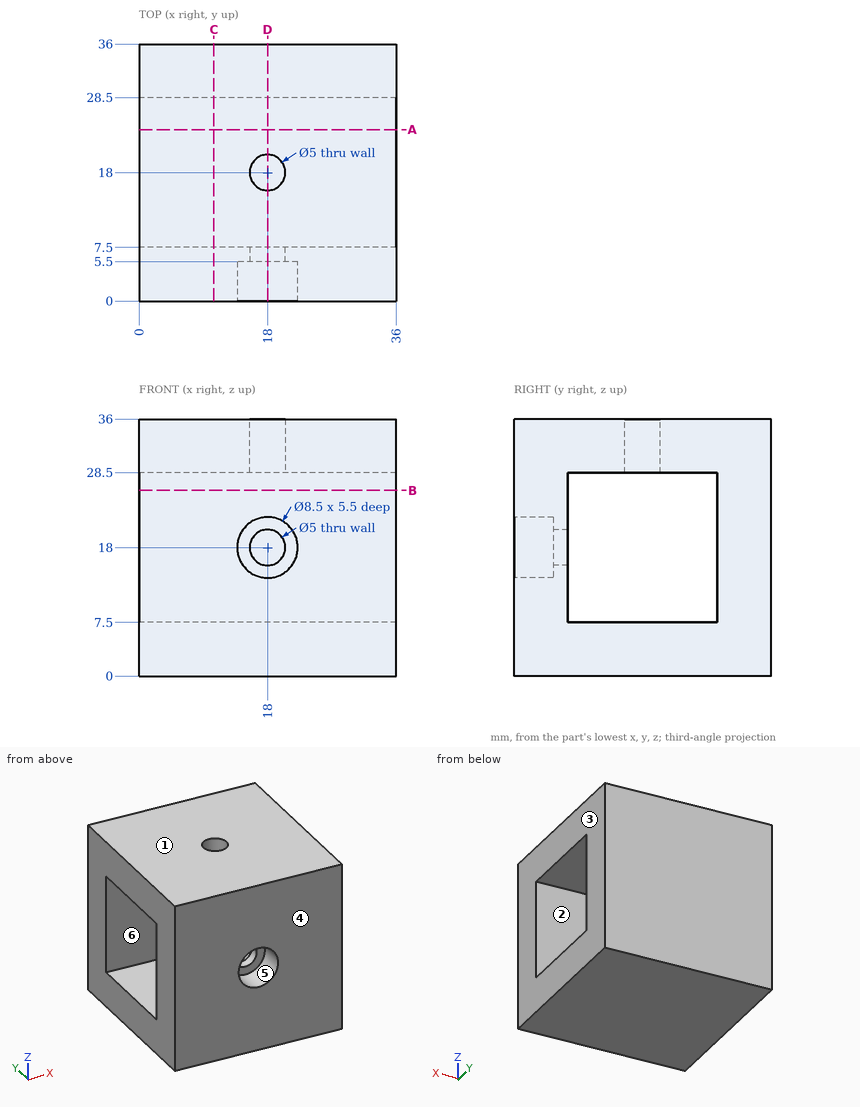
Design review of the part shown in the three views and the two pictorial views. Dimensions are in mm from the part's minimum x, y and z. A direction names the side the tool comes from. Give positions to 0.01 mm unless a question says otherwise; leave off trailing zeros. Write each loop counter-clockwise with the first axis right and the second up, starting at its lowest first coordinate (ties: lowest second). Pieces come first, ordered by that corner, then holes. Notation, with made-up numbers: (-1.75, 50.5) -> (10.25, 50.5) arc R5 ccw to (10.25, 54.5) -> close; hole circle Ø5 at (28.5, 68). An arc over 180 degrees is marked (long way). Answer in a Markdown table with one row per item.
1) Tool access review of the marked faces 4, 5 and 6: name each direction out of +Z, -Z, +X, -X, +Y, -Y from which nothing blocks a thin tool from reaching the whole face with its end or side.
Worked answers:
| item | result |
|---|---|
| face 4 | +Z, -Z, +X, -X, -Y |
| face 5 | -Y |
| face 6 | +X, -X |
2) Mouldability with a two-part tool opening along Z and no side actions: class the marked faces 1, 2 and 3 as +Z half, -Z half, draft (parallel to the pull), parting line (faces both ways), or undercut.
Worked answers:
| item | result |
|---|---|
| face 1 | +Z half |
| face 2 | undercut |
| face 3 | draft |
3) Add section C-C on x = 10.5. State the section outline as (y, z) points.
Worked answers:
| item | result |
|---|---|
| outline | (0, 0) -> (36, 0) -> (36, 36) -> (0, 36) -> close; hole (7.5, 7.5) -> (28.5, 7.5) -> (28.5, 28.5) -> (7.5, 28.5) -> close |
4) For L1, parallel to Z at x = 25, y = 19.5; L2, parallel to Z at x = 18, y = 6.85, list the stretches that pass through material, from the lowest coordinate up. Write a range as [from, to].
Worked answers:
| item | result |
|---|---|
| L1 | [0, 7.5], [28.5, 36] |
| L2 | [0, 15.5], [20.5, 36] |
5) Clearance check with flat-ended pins moving along their axes: P1, Ø3, axis at y = 26.5, z = 7.5, coming from the -X side; P2, Ø3, axis at x = 18, y = 18, coming from the +Z side; P3, Ø7, axis at x = 18.5, z = 18, coming from the -Y side. State where each tip first meets the part, or that it passes through.
Worked answers:
| item | result |
|---|---|
| P1 | x = 0 |
| P2 | z = 7.5 |
| P3 | y = 5.5 |
6) Add section D-D on x = 18. State the section outline as (y, z) points.
Worked answers:
| item | result |
|---|---|
| outline | (0, 0) -> (36, 0) -> (36, 36) -> (20.5, 36) -> (20.5, 28.5) -> (28.5, 28.5) -> (28.5, 7.5) -> (7.5, 7.5) -> (7.5, 15.5) -> (5.5, 15.5) -> (5.5, 13.75) -> (0, 13.75) -> close; (0, 22.25) -> (5.5, 22.25) -> (5.5, 20.5) -> (7.5, 20.5) -> (7.5, 28.5) -> (15.5, 28.5) -> (15.5, 36) -> (0, 36) -> close |
7) Add section A-A on y = 24. State the section outline as (x, z) points.
Worked answers:
| item | result |
|---|---|
| outline | (0, 0) -> (36, 0) -> (36, 7.5) -> (0, 7.5) -> close; (0, 28.5) -> (36, 28.5) -> (36, 36) -> (0, 36) -> close |
